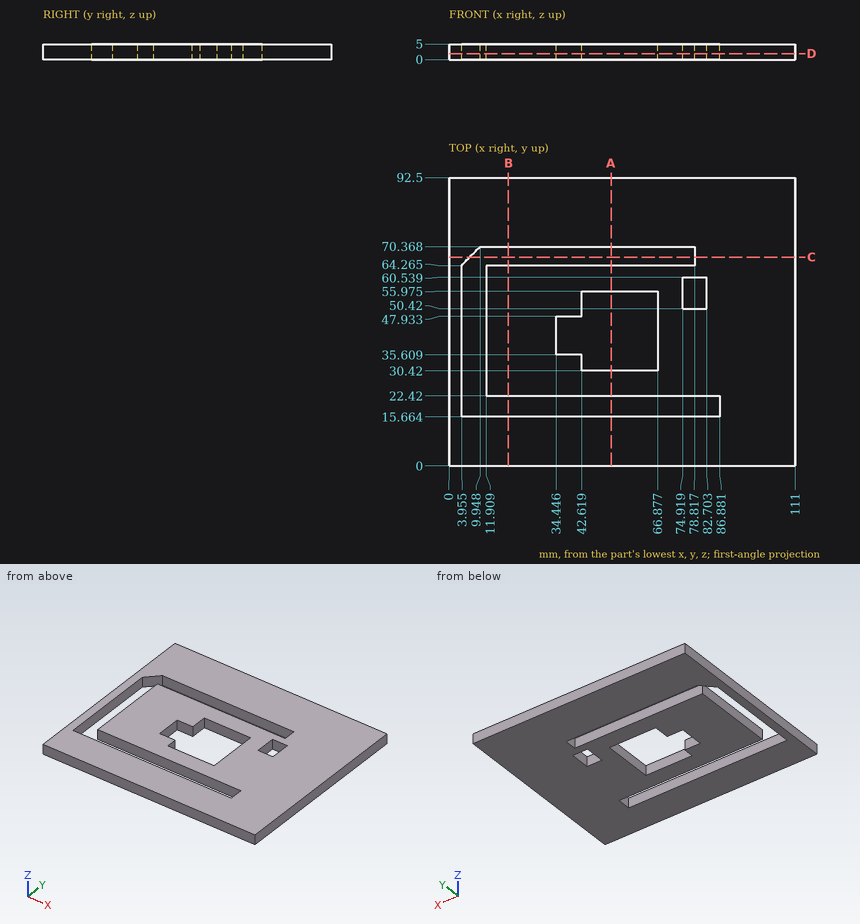
Geometry check sheet. Reference: drawing and pictorial views, mm from the part's lowest x, y, z. Round coordinates to 2 decimals unless told otherwise and drop trailing zeros. Write each loop counter-clockwise with the first axis right and the second up, starting at its lowest first coordinate (ties: lowest second). Pieces come first, ordered by that corner, then holes. Notation, with made-up numbers: (43, 57.25) -> (75, 57.25) arc R19 ccw to (75, 87.25) -> close; hole circle Ø2 at (25.5, 2.25). An arc over 180 degrees is marked (long way). Put each result on its own line as item: value.
1) Cross-section at B-B, the plane x = 19. Enter the section's corners in (y, z) (1 decimal), plus the area to 3 significant figures.
Recorded:
outline: (0, 0) -> (15.7, 0) -> (15.7, 5) -> (0, 5) -> close; (22.4, 0) -> (64.3, 0) -> (64.3, 5) -> (22.4, 5) -> close; (70.4, 0) -> (92.5, 0) -> (92.5, 5) -> (70.4, 5) -> close
area: 398 mm2
2) Cross-section at C-C, the plane y = 67. Enter the section's corners in (x, z), plus the area to 3 significant figures.
Recorded:
outline: (0, 0) -> (6.64, 0) -> (6.64, 5) -> (0, 5) -> close; (78.82, 0) -> (111, 0) -> (111, 5) -> (78.82, 5) -> close
area: 194 mm2
3) Cross-section at A-A, the plane x = 52. Enter the section's corners in (y, z) (1 decimal).
Recorded:
outline: (0, 0) -> (15.7, 0) -> (15.7, 5) -> (0, 5) -> close; (22.4, 0) -> (30.4, 0) -> (30.4, 5) -> (22.4, 5) -> close; (56, 0) -> (64.3, 0) -> (64.3, 5) -> (56, 5) -> close; (70.4, 0) -> (92.5, 0) -> (92.5, 5) -> (70.4, 5) -> close
4) Cross-section at D-D, the plane z = 1.9. Enter the section's corners in (x, y) (1 decimal).
Recorded:
outline: (0, 0) -> (111, 0) -> (111, 92.5) -> (0, 92.5) -> close; hole (4, 15.7) -> (86.9, 15.7) -> (86.9, 22.4) -> (11.9, 22.4) -> (11.9, 64.3) -> (78.8, 64.3) -> (78.8, 70.4) -> (9.9, 70.4) -> (4, 64.3) -> close; hole (34.4, 35.6) -> (42.6, 35.6) -> (42.6, 30.4) -> (66.9, 30.4) -> (66.9, 56) -> (42.6, 56) -> (42.6, 47.9) -> (34.4, 47.9) -> close; hole (74.9, 50.4) -> (82.7, 50.4) -> (82.7, 60.5) -> (74.9, 60.5) -> close
5) Thickness scan on probe 1 along Y at (x, z) = (66, 3.25) (1 decimal); probe 2 along Y at (x, z) = (35, 3.95) (1 decimal); probe 3 along X at (y, z) = (59.5, 4.5) (1 decimal). Record the ranges inside material, lowest first. Write a range as from..to.
Recorded:
probe 1: y = 0..15.7, 22.4..30.4, 56..64.3, 70.4..92.5
probe 2: y = 0..15.7, 22.4..35.6, 47.9..64.3, 70.4..92.5
probe 3: x = 0..4, 11.9..74.9, 82.7..111
